Geometry: final body of the model. Coordinates: model frame, mm. A direction names the side the tool comes from. Round coordinates to 2 decimals unless told otherwise and drop trailing zeros. Loops run counter-clockwise (first coordinate to the right, second up) from the corner with the lowest first, then second, coordinate; pieces in that order, holes last. Notation, with made-up numbers: (-29, -17) - (1, -17) arc R23 cw to (1, 19) - close; hole circle Ø10 at (48, -33). An arc over 180 degrees is marked (long way). Write item = value, one per line. Start each with the question number.
Item 1: Section B-B (y = 1). Return loops of the section in (x, z), plus the area to 3 significant figures.
Item 2: Access query for faces 4 (the flat face through (2.1, 1, 6)), 5 (the flat face through (-23, 6, 15)), 6 (the flat face through (-23, 6, -15)), 7 (the cylindrical face through (-10.81, 1.63, -34.34)). Directions: +Z, -Z, +X, -X, +Y, -Y. A direction counts if a zero-diameter tool reaches every point of the face in a straight line with its end or side. Return the directions, or none.
Item 3: Line query: line 1 (X direction, y = 7.5, z = 4.5); line 2 (Y direction, x = 22.5, z = 17.5); line 3 (X direction, y = 4, z = 7). Output: solid intervals per line, ascending. Write a range as from..to.
Item 4: Section A-A (y = 6.5). Return loops of the section in (x, z), plus the area to 3 significant figures.
Item 5: Draft query along X for faces 1 (the flat face through (25, 6, 0)), 2 (the flat face through (23, 6, -15)), 3 (the cylindrical face through (0.05, 1.48, -9.75)). Return one class per face: pulls with the +X half, pulls with the -X half, needs draft (parallel to the pull), parting line crosses it, or undercut.
Item 6: First-contact query: pin 1 (0.8 mm diameter, centred on x = -16, z = 0, fed in from +Y); pin 2 (3 mm diameter, centred on y = 1.5, z = 9.5, fed in from -X); pin 3 (2 mm diameter, centred on y = 4, z = -5, fed in from -X); pin 4 (1.5 mm diameter, centred on x = -27.5, z = -23, fed in from -Y). Flat tips, straight axial feed; report the tip coordinate or a pass-through.
from build123d import *

# Parameters (mm, degrees)
CROQUIS1_R              = 36
CROQUIS1_R_2            = 1.75
SALIENTE_EXTRUIR1_DEPTH = 4.3
CROQUIS2_W              = 4.5
CROQUIS2_H              = 30
SALIENTE_EXTRUIR2_DEPTH = 4.3
REDONDEO1_R             = 1
CORTAR_EXTRUIR1_DEPTH   = 3
CROQUIS4_R              = 1.75
CORTAR_EXTRUIR2_DEPTH   = 10
CROQUIS5_R              = 0.65
CORTAR_EXTRUIR3_DEPTH   = 10


with BuildPart() as part:
    # Croquis1 → Saliente-Extruir1 (new body)
    with BuildSketch(Plane(origin=(0, 0, 0), x_dir=(1, 0, 0), z_dir=(0, 1, 0))):
        with Locations(Location((0, 0, 0), (0, 0, 90))):
            Circle(CROQUIS1_R)
        with Locations(Location((0, 14, 0), (0, 0, 90))):
            Circle(CROQUIS1_R_2, mode=Mode.SUBTRACT)
        with Locations(Location((0, -14, 0), (0, 0, 90))):
            Circle(CROQUIS1_R_2, mode=Mode.SUBTRACT)
    extrude(amount=SALIENTE_EXTRUIR1_DEPTH)

    # Croquis2 → Saliente-Extruir2 (add)
    with BuildSketch(Plane(origin=(0, 4.3, 0), x_dir=(1, 0, 0), z_dir=(0, 1, 0))):
        with Locations((22.75, 0)):
            Rectangle(CROQUIS2_W, CROQUIS2_H)
        with Locations((-22.75, 0)):
            Rectangle(CROQUIS2_W, CROQUIS2_H)
    extrude(amount=SALIENTE_EXTRUIR2_DEPTH)

    # Redondeo1
    redondeo1_edges = [part.edges().sort_by_distance(p)[0] for p in [
        (25, 4.3, 0),
        (25, 8.6, 0),
        (-25, 4.3, 0),
        (-25, 8.6, 0),
        (0, 4.3, 36),
    ]]
    fillet(redondeo1_edges, radius=REDONDEO1_R)

    # Croquis3 → Cortar-Extruir1 (cut)
    with BuildSketch(Plane.XZ):
        with BuildLine():
            Line((2.1, 3.659676792), (16.8, 2.5))
            ThreePointArc((16.8, 2.5), (19.3, 0), (16.8, -2.5))
            Line((16.8, -2.5), (2.1, -3.659676792))
            Line((2.1, -3.659676792), (2.1, -7.65))
            ThreePointArc((2.1, -7.65), (0, -9.75), (-2.1, -7.65))
            Line((-2.1, -7.65), (-2.1, -3.659676792))
            Line((-2.1, -3.659676792), (-16.8, -2.5))
            ThreePointArc((-16.8, -2.5), (-19.3, 0), (-16.8, 2.5))
            Line((-16.8, 2.5), (-2.1, 3.659676792))
            Line((-2.1, 3.659676792), (-2.1, 7.65))
            ThreePointArc((-2.1, 7.65), (0, 9.75), (2.1, 7.65))
            Line((2.1, 7.65), (2.1, 3.659676792))
        make_face()
    extrude(amount=-CORTAR_EXTRUIR1_DEPTH, mode=Mode.SUBTRACT)

    # Croquis4 → Cortar-Extruir2 (cut)
    with BuildSketch(Plane.XZ):
        with Locations(Location((0, 0, 0), (0, 0, 270))):
            Circle(CROQUIS4_R)
    extrude(amount=-CORTAR_EXTRUIR2_DEPTH, mode=Mode.SUBTRACT)

    # Croquis5 → Cortar-Extruir3 (cut)
    with BuildSketch(Plane.XZ):
        with Locations(Location((16, 0, 0), (0, 0, 270))):
            Circle(CROQUIS5_R)
        with Locations(Location((-16, 0, 0), (0, 0, 270))):
            Circle(CROQUIS5_R)
        with Locations(Location((0, 7.5, 0), (0, 0, 270))):
            Circle(CROQUIS5_R)
        with Locations(Location((0, -7.5, 0), (0, 0, 270))):
            Circle(CROQUIS5_R)
    extrude(amount=-CORTAR_EXTRUIR3_DEPTH, mode=Mode.SUBTRACT)


solid = part.part
Taken from the geometry:
q1.outline = circle Ø72 at (0, 0); hole (-16.8, -2.5) - (-2.1, -3.66) - (-2.1, -7.65) arc R2.1 ccw to (2.1, -7.65) - (2.1, -3.66) - (16.8, -2.5) arc R2.5 ccw to (16.8, 2.5) - (2.1, 3.66) - (2.1, 7.65) arc R2.1 ccw to (-2.1, 7.65) - (-2.1, 3.66) - (-16.8, 2.5) arc R2.5 ccw to start; hole circle Ø3.5 at (0, -14); hole circle Ø3.5 at (0, 14)
q1.area = 3,770 mm^2
q2.face_4 = -Y
q2.face_5 = +Z, +X, -X, +Y
q2.face_6 = -Z, +X, -X, +Y
q2.face_7 = +Y, -Y
q3.line_1 = -25..-20.5, 20.5..25
q3.line_2 = 0..4.3
q3.line_3 = -35.02..-0.42, 0.42..35.02
q4.outline = (-25, -15) - (-20.5, -15) - (-20.5, 15) - (-25, 15) - close; (20.5, -15) - (25, -15) - (25, 15) - (20.5, 15) - close
q4.area = 270 mm^2
q5.face_1 = pulls with the +X half
q5.face_2 = needs draft
q5.face_3 = undercut
q6.pin_1 = through
q6.pin_2 = -35.1
q6.pin_3 = -35.75
q6.pin_4 = 0
